Build history of the part. All positions in model axes, mm. Face numbers are marked on the shaded views. A direction names the side the tool comes from. Round coordinates to 2 decimals unless told otherwise and drop trailing zeros. Loops run counter-clockwise (first coordinate to the right, second up) from the corner with the lowest first, then second, coordinate; pieces in that order, holes last. Notation, with made-up numbers: (9, 70.5) - (49, 70.5) arc R19 cw to (49, 89.5) - close; hole circle Ø6 at (30.25, -10). An arc over 180 degrees is marked (long way). Use a Markdown table: item, result.
from build123d import *
from OCP.BRepFilletAPI import BRepFilletAPI_MakeChamfer

# Parameters (mm, degrees)
EXTRUDE_1_DEPTH     = 6
CUT_EXTRUDE_1_DEPTH = 2.1
CUT_EXTRUDE_2_DEPTH = 4
SKETCH_3_W          = 86
SKETCH_3_H          = 2
EXTRUDE_2_DEPTH     = 2
SKETCH_4_W          = 2
SKETCH_4_H          = 10
EXTRUDE_3_DEPTH     = 4
FILLET_1_R          = 1
CHAMFER_1_SIZE      = 1
CHAMFER_1_SIZE2     = 1.732050808
CHAMFER_2_SIZE      = 0.4
CHAMFER_2_SIZE2     = 0.692820323
SKETCH_5_R          = 1.2
CUT_EXTRUDE_3_DEPTH = 45.481569217
SKETCH_5_3_R        = 2.05
CUT_EXTRUDE_4_DEPTH = 2
CHAMFER_3_SIZE      = 0.2
CHAMFER_3_SIZE2     = 0.346410162


with BuildPart() as part:
    # 草图1 → 凸台-拉伸1 (new body)
    with BuildSketch(Plane(origin=(0, 0, 0), x_dir=(1, 0, 0), z_dir=(0, 1, 0))):
        Polygon((-43, 2), (-33.15, 2), (-33.15, 4.1), (-34.95, 5.9), (-34.95, 6.1), (-27.35, 6.1), (-27.35, 5.9), (-29.15, 4.1), (-29.15, 2), (29.15, 2), (29.15, 4.1), (27.35, 5.9), (27.35, 6.1), (34.95, 6.1), (34.95, 5.9), (33.15, 4.1), (33.15, 2), (43, 2), (43, -2), (-43, -2), align=None)
    extrude(amount=EXTRUDE_1_DEPTH)

    # 草图2 → 切除-拉伸1 (cut)
    with BuildSketch(Plane(origin=(0, 0, -2), x_dir=(-1, 0, 0), z_dir=(0, 0, -1))):
        with BuildLine():
            Line((-15.5, 5.25), (15.5, 5.25))
            ThreePointArc((15.5, 5.25), (17.75, 3), (15.5, 0.75))
            Line((15.5, 0.75), (-15.5, 0.75))
            ThreePointArc((-15.5, 0.75), (-17.75, 3), (-15.5, 5.25))
        make_face()
    extrude(amount=-CUT_EXTRUDE_1_DEPTH, mode=Mode.SUBTRACT)

    # 草图2<3> → 切除-拉伸2 (cut)
    with BuildSketch(Plane(origin=(0, 0, -2), x_dir=(-1, 0, 0), z_dir=(0, 0, -1))):
        with BuildLine():
            Line((-12.3, 5.25), (12.3, 5.25))
            ThreePointArc((12.3, 5.25), (14.55, 3), (12.3, 0.75))
            Line((12.3, 0.75), (-12.3, 0.75))
            ThreePointArc((-12.3, 0.75), (-14.55, 3), (-12.3, 5.25))
        make_face()
    extrude(amount=-CUT_EXTRUDE_2_DEPTH, mode=Mode.SUBTRACT)

    # 草图3 → 凸台-拉伸2 (add)
    with BuildSketch(Plane.XY.offset(2)):
        with Locations((0, 7)):
            Rectangle(SKETCH_3_W, SKETCH_3_H)
        with Locations((0, -1)):
            Rectangle(SKETCH_3_W, SKETCH_3_H)
    extrude(amount=-EXTRUDE_2_DEPTH)

    # 草图4 → 凸台-拉伸3 (add)
    with BuildSketch(Plane.XY.offset(2)):
        with Locations((42, 3)):
            Rectangle(SKETCH_4_W, SKETCH_4_H)
    extrude(amount=-EXTRUDE_3_DEPTH)

    # 圆角1
    fillet_1_edges = [part.edges().sort_by_distance(p)[0] for p in [
        (43, -2, 0),
        (43, 8, 0),
    ]]
    fillet(fillet_1_edges, radius=FILLET_1_R)

    # 倒角1
    chamfer_1_edges = [part.edges().sort_by_distance(p)[0] for p in [
        (-43, 3, 2),
    ]]
    chamfer_1_side = [part.faces().sort_by_distance(p)[0] for p in [
        (-43, 3, 0.25),
    ]]
    chamfer(chamfer_1_edges, length=CHAMFER_1_SIZE, length2=CHAMFER_1_SIZE2, reference=chamfer_1_side[0])

    # 倒角2: one chamfer whose edges measure the first distance from different faces: ONE call of the kernel's chamfer builder (chamfer() names one face for all edges)
    chamfer_2_edges_1 = [part.edges().sort_by_distance(p)[0] for p in [
        (-1, -2, 0),
    ]]
    chamfer_2_side_1 = [part.faces().sort_by_distance(p)[0] for p in [
        (-1, -1, 0),
    ]]
    chamfer_2_edges_2 = [part.edges().sort_by_distance(p)[0] for p in [
        (-1, 8, 0),
    ]]
    chamfer_2_side_2 = [part.faces().sort_by_distance(p)[0] for p in [
        (-1, 7, 0),
    ]]
    chamfer_2_edges_3 = [part.edges().sort_by_distance(p)[0] for p in [
        (43, 3, 2),
    ]]
    chamfer_2_side_3 = [part.faces().sort_by_distance(p)[0] for p in [
        (43, 3, 0),
    ]]
    chamfer_2_edges_4 = [part.edges().sort_by_distance(p)[0] for p in [
        (0.366025404, 8, 2),
    ]]
    chamfer_2_side_4 = [part.faces().sort_by_distance(p)[0] for p in [
        (0.202993546, 8, 0.973252826),
    ]]
    chamfer_2_edges_5 = [part.edges().sort_by_distance(p)[0] for p in [
        (42.707106781, 7.707106781, 2),
    ]]
    chamfer_2_side_5 = [part.faces().sort_by_distance(p)[0] for p in [
        (42.707106781, 7.707106781, 0),
    ]]
    chamfer_2_edges_6 = [part.edges().sort_by_distance(p)[0] for p in [
        (42.707106781, -1.707106781, 2),
    ]]
    chamfer_2_side_6 = [part.faces().sort_by_distance(p)[0] for p in [
        (42.707106781, -1.707106781, 0),
    ]]
    chamfer_2_edges_7 = [part.edges().sort_by_distance(p)[0] for p in [
        (0.366025404, -2, 2),
    ]]
    chamfer_2_side_7 = [part.faces().sort_by_distance(p)[0] for p in [
        (0.202993546, -2, 0.973252826),
    ]]
    chamfer_2 = BRepFilletAPI_MakeChamfer(part.part.solid().wrapped)
    for e in chamfer_2_edges_1:
        chamfer_2.Add(CHAMFER_2_SIZE, CHAMFER_2_SIZE2, e.wrapped, chamfer_2_side_1[0].wrapped)  # the first distance lies on this face
    for e in chamfer_2_edges_2:
        chamfer_2.Add(CHAMFER_2_SIZE, CHAMFER_2_SIZE2, e.wrapped, chamfer_2_side_2[0].wrapped)  # the first distance lies on this face
    for e in chamfer_2_edges_3:
        chamfer_2.Add(CHAMFER_2_SIZE, CHAMFER_2_SIZE2, e.wrapped, chamfer_2_side_3[0].wrapped)  # the first distance lies on this face
    for e in chamfer_2_edges_4:
        chamfer_2.Add(CHAMFER_2_SIZE, CHAMFER_2_SIZE2, e.wrapped, chamfer_2_side_4[0].wrapped)  # the first distance lies on this face
    for e in chamfer_2_edges_5:
        chamfer_2.Add(CHAMFER_2_SIZE, CHAMFER_2_SIZE2, e.wrapped, chamfer_2_side_5[0].wrapped)  # the first distance lies on this face
    for e in chamfer_2_edges_6:
        chamfer_2.Add(CHAMFER_2_SIZE, CHAMFER_2_SIZE2, e.wrapped, chamfer_2_side_6[0].wrapped)  # the first distance lies on this face
    for e in chamfer_2_edges_7:
        chamfer_2.Add(CHAMFER_2_SIZE, CHAMFER_2_SIZE2, e.wrapped, chamfer_2_side_7[0].wrapped)  # the first distance lies on this face
    add(Compound.cast(chamfer_2.Shape()), mode=Mode.REPLACE)

    # 草图5 → 切除-拉伸3 (cut, through all)
    with BuildSketch(Plane.XY.offset(2)):
        with Locations((38, 3)):
            Circle(SKETCH_5_R)
    extrude(amount=-CUT_EXTRUDE_3_DEPTH, mode=Mode.SUBTRACT)

    # 草图5<3> → 切除-拉伸4 (cut)
    with BuildSketch(Plane.XY.offset(2)):
        with Locations((38, 3)):
            Circle(SKETCH_5_3_R)
    extrude(amount=-CUT_EXTRUDE_4_DEPTH, mode=Mode.SUBTRACT)

    # 倒角3: one chamfer whose edges measure the first distance from different faces: ONE call of the kernel's chamfer builder (chamfer() names one face for all edges)
    chamfer_3_edges_1 = [part.edges().sort_by_distance(p)[0] for p in [
        (-43, -0.8, 0),
    ]]
    chamfer_3_side_1 = [part.faces().sort_by_distance(p)[0] for p in [
        (-1, -0.8, 0),
    ]]
    chamfer_3_edges_2 = [part.edges().sort_by_distance(p)[0] for p in [
        (-43, 6.8, 0),
    ]]
    chamfer_3_side_2 = [part.faces().sort_by_distance(p)[0] for p in [
        (-1, 6.8, 0),
    ]]
    chamfer_3 = BRepFilletAPI_MakeChamfer(part.part.solid().wrapped)
    for e in chamfer_3_edges_1:
        chamfer_3.Add(CHAMFER_3_SIZE, CHAMFER_3_SIZE2, e.wrapped, chamfer_3_side_1[0].wrapped)  # the first distance lies on this face
    for e in chamfer_3_edges_2:
        chamfer_3.Add(CHAMFER_3_SIZE, CHAMFER_3_SIZE2, e.wrapped, chamfer_3_side_2[0].wrapped)  # the first distance lies on this face
    add(Compound.cast(chamfer_3.Shape()), mode=Mode.REPLACE)


solid = part.part
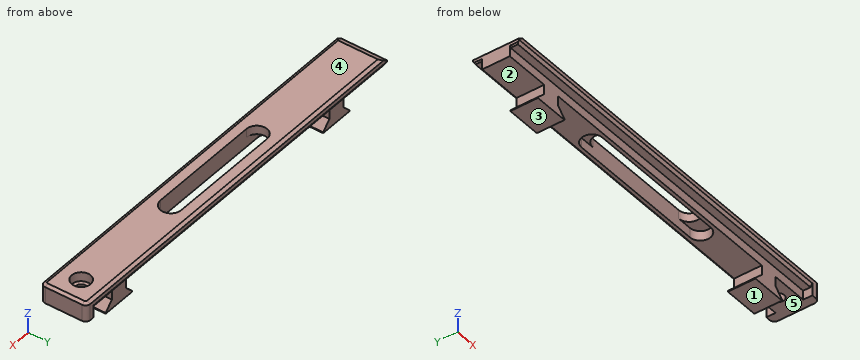
Q1. Cut at B-B, the plane x = 38. List the corners of the cut face in (y, z), plus the area to 3 significant figures.
Results found:
| item | result |
|---|---|
| outline | (-2, 0.69) - (-1.6, 0) - (0, 0) - (0, -2) - (1.8, -2) - (1.8, 0) - (0.95, 0) - (0.95, 2) - (-1.31, 2) - (-2, 1.6) - close; (4.2, -2) - (6, -2) - (6, 0) - (7.6, 0) - (8, 0.69) - (8, 1.6) - (7.31, 2) - (5.05, 2) - (5.05, 0) - (4.2, 0) - close |
| area | 18.4 mm2 |
Q2. Drop flat-ended pins along their axis: pin 1 (0.8 mm diameter, centred on x = 14, y = -1, fed in from -Z); pin 2 (1.5 mm diameter, centred on x = -3, y = 0.5, fed in from -Z); pin 3 (4 mm diameter, centred on x = 38, y = 3, fed in from +Z). Give the stop position or say it passes through.
Results found:
| item | result |
|---|---|
| pin 1 | stops at z = 0 |
| pin 2 | stops at z = -2 |
| pin 3 | stops at z = 0 |
Q3. Probe line 1 (Y direction, x = 38, z = 1.5); line 2 (Y direction, x = 38, z = -0.45); line 3 (Y direction, x = 33, z = -2.25). List the from-to ranges inside material, lowest first.
Results found:
| item | result |
|---|---|
| line 1 | y = -2 to 0.95, 5.05 to 8 |
| line 2 | y = 0 to 1.8, 4.2 to 6 |
| line 3 | y = 0 to 6 |
Q4. Which spindle directions (+Z, -Z, +X, -X, +Y, -Y) get a long thin tool onto all of the face, cutting with end or side? Do the marked faces 1 and 2. Say none if no direction does.
Results found:
| item | result |
|---|---|
| face 1 | -Z, +X, -X, +Y, -Y |
| face 2 | -X, +Y, -Y |
Q5. Cut at D-D, the plane x = 13.5. List the corners of the cut face in (y, z).
Results found:
| item | result |
|---|---|
| outline | (-2, 0.69) - (-1.6, 0) - (0, 0) - (0, -2) - (0.75, -2) - (0.75, 0.1) - (1.1, 0.1) - (1.1, 2) - (-1.31, 2) - (-2, 1.6) - close; (4.9, 0.1) - (5.25, 0.1) - (5.25, -2) - (6, -2) - (6, 0) - (7.6, 0) - (8, 0.69) - (8, 1.6) - (7.31, 2) - (4.9, 2) - close |
Q6. Cut at A-A, the plane x = -1. List the corners of the cut face in (y, z).
Results found:
| item | result |
|---|---|
| outline | (-2, 0.69) - (-1.6, 0) - (0, 0) - (0, -2) - (0.75, -2) - (0.75, 2) - (-1.31, 2) - (-2, 1.6) - close; (5.25, -2) - (6, -2) - (6, 0) - (7.6, 0) - (8, 0.69) - (8, 1.6) - (7.31, 2) - (5.25, 2) - close |
Q7. Cut at C-C, the plane y = 3. Count the separate pieces of the cut face and the enclosed holes in it, plus the area to 3 significant figures.
Results found:
| item | result |
|---|---|
| separate pieces | 3 |
| enclosed holes | 0 |
| area | 241 mm2 |
Q8. Pull direction Z, two halves, no side cores. Call the marked faces 3, 4 and 5: pulls with the +Z half, pulls with the -Z half, needs draft (parallel to the pull), parting line crosses it, or undercut.
Results found:
| item | result |
|---|---|
| face 3 | pulls with the -Z half |
| face 4 | pulls with the +Z half |
| face 5 | undercut |
